from build123d import *

# Parameters (mm, degrees)
BOSS_EXTRUDE2_DEPTH          = 12
BOSS_EXTRUDE3_START          = -2
BOSS_EXTRUDE3_DEPTH          = 10
BOSS_EXTRUDE4_START          = 10
BOSS_EXTRUDE4_DEPTH          = 22
BOSS_EXTRUDE7_DEPTH          = 40
BOSS_EXTRUDE17_DEPTH         = 6
BOSS_EXTRUDE17_DEPTH_BACK    = 6
CUT_EXTRUDE_THIN1_DEPTH      = 297.279628574
CUT_EXTRUDE_THIN1_DEPTH_BACK = 297.279628574
CUT_EXTRUDE1_START           = -8
SKETCH6_R                    = 5
CUT_EXTRUDE1_DEPTH           = 231.29743947
SKETCH6_4_R                  = 2.75
CUT_EXTRUDE2_DEPTH           = 239.29743947


with BuildPart() as part:
    # Sketch2 → Boss-Extrude2 (new body)
    with BuildSketch(Plane(origin=(0, 0, 0), x_dir=(1, 0, 0), z_dir=(0, 1, 0))):
        with BuildLine():
            Line((-292.596610314, 15.743442535), (-276.02456554, 0))
            Line((-276.02456554, 0), (-292.596610314, -17.444257657))
            Line((-292.596610314, -17.444257657), (-286.510767905, -23.850407561))
            Line((-286.510767905, -23.850407561), (-256.02456554, -12.789688675))
            Line((-256.02456554, -12.789688675), (0.21086679, -12.5))
            ThreePointArc((0.21086679, -12.5), (0.401744327, -17.25142014), (0.653571446, -22))
            Line((0.653571446, -22), (6.263616969, -22))
            ThreePointArc((6.263616969, -22), (5.6, 0), (6.263616969, 22))
            Line((6.263616969, 22), (0.653571446, 22))
            ThreePointArc((0.653571446, 22), (0.401744327, 17.25142014), (0.21086679, 12.5))
            Line((0.21086679, 12.5), (-256.02456554, 12.210311325))
            Line((-256.02456554, 12.210311325), (-286.510767905, 22.149592439))
            Line((-286.510767905, 22.149592439), (-292.596610314, 15.743442535))
        make_face()
    extrude(amount=-BOSS_EXTRUDE2_DEPTH)

    # Sketch2<5> → Boss-Extrude3 (add)
    with BuildSketch(Plane(origin=(0, 0, 0), x_dir=(1, 0, 0), z_dir=(0, 1, 0)).offset(BOSS_EXTRUDE3_START)):
        with BuildLine():
            Line((25.340211435, 22), (6.263616969, 22))
            ThreePointArc((6.263616969, 22), (5.6, 0), (6.263616969, -22))
            Line((6.263616969, -22), (25.340211435, -22))
            ThreePointArc((25.340211435, -22), (24.64, 0), (25.340211435, 22))
        make_face()
    extrude(amount=-BOSS_EXTRUDE3_DEPTH)

    # Sketch2<6> → Boss-Extrude4 (add)
    with BuildSketch(Plane(origin=(0, 0, 0), x_dir=(1, 0, 0), z_dir=(0, 1, 0)).offset(BOSS_EXTRUDE4_START)):
        with BuildLine():
            ThreePointArc((0.653571446, 22), (0.401744327, 17.25142014), (0.21086679, 12.5))
            ThreePointArc((0.21086679, 12.5), (0, 0), (0.21086679, -12.5))
            ThreePointArc((0.21086679, -12.5), (0.401744327, -17.25142014), (0.653571446, -22))
            Line((0.653571446, -22), (6.263616969, -22))
            ThreePointArc((6.263616969, -22), (5.6, 0), (6.263616969, 22))
            Line((6.263616969, 22), (0.653571446, 22))
        make_face()
    extrude(amount=-BOSS_EXTRUDE4_DEPTH)

    # Sketch2<9> → Boss-Extrude7 (add)
    with BuildSketch(Plane(origin=(0, 0, 0), x_dir=(1, 0, 0), z_dir=(0, 1, 0))):
        Polygon((-292.596610314, 15.743442535), (-276.02456554, 0), (-292.596610314, -17.444257657), (-286.510767905, -23.850407561), (-219.731467486, 0.377833809), (-286.510767905, 22.149592439), align=None)
    extrude(amount=BOSS_EXTRUDE7_DEPTH)

    # Sketch4 → Boss-Extrude17 (add, two sides: drawn at the far end of the back side and taken through both)
    with BuildSketch(Plane.XY.offset(-BOSS_EXTRUDE17_DEPTH_BACK)):
        Polygon((0.653571446, 10), (-256.02456554, 40), (-256.02456554, 0), (0.653571446, 0), align=None)
    extrude(amount=BOSS_EXTRUDE17_DEPTH + BOSS_EXTRUDE17_DEPTH_BACK)

    # Sketch5 → Cut-Extrude-Thin1 (cut, two sides: drawn at the far end of the back side and taken through both)
    with BuildSketch(Plane.XY.offset(-CUT_EXTRUDE_THIN1_DEPTH_BACK)):
        Polygon((0.653571446, 10), (-256.02456554, 40), (-254.863688753, 49.932389697), (1.814448233, 19.932389697), align=None)
    extrude(amount=CUT_EXTRUDE_THIN1_DEPTH + CUT_EXTRUDE_THIN1_DEPTH_BACK, mode=Mode.SUBTRACT)

    # Sketch6 → Cut-Extrude1 (cut, through all)
    with BuildSketch(Plane(origin=(-145.085185566, 0, -137.830926288), x_dir=(-0.6887494619146907, 0, 0.724999433594416), z_dir=(-0.724999433594416, 0, -0.6887494619146907)).offset(CUT_EXTRUDE1_START)):
        with Locations((200.111770991, 29)):
            Circle(SKETCH6_R)
        with Locations((200.111770991, -1)):
            Circle(SKETCH6_R)
    cut_extrude1 = extrude(amount=-CUT_EXTRUDE1_DEPTH, mode=Mode.SUBTRACT)

    # Sketch6<4> → Cut-Extrude2 (cut, symmetric)
    with BuildSketch(Plane(origin=(-145.085185566, 0, -137.830926288), x_dir=(-0.6887494619146907, 0, 0.724999433594416), z_dir=(-0.724999433594416, 0, -0.6887494619146907))):
        with Locations((200.111770991, 29)):
            Circle(SKETCH6_4_R)
        with Locations((200.111770991, -1)):
            Circle(SKETCH6_4_R)
    cut_extrude2 = extrude(amount=CUT_EXTRUDE2_DEPTH, both=True, mode=Mode.SUBTRACT)

    # Mirror1: Cut-Extrude1, Cut-Extrude2 across plane
    add(cut_extrude1.mirror(Plane.XY), mode=Mode.SUBTRACT)
    add(cut_extrude2.mirror(Plane.XY), mode=Mode.SUBTRACT)


solid = part.part
CAD build for the part. Positions are in the model's coordinates, mm. A direction names the side the tool comes from. Coordinates: 2 decimals unless noted, no trailing zeros. Loops run counter-clockwise (first coordinate to the right, second up) from the corner with the lowest first, then second, coordinate; pieces in that order, holes last. Notation, with made-up numbers: (8.25, 5) - (66.25, 5) arc R14 cw to (66.25, 21) - close; hole circle Ø11 at (-25.5, 24). An arc over 180 degrees is marked (long way). Write item = value, one per line. Start each with the question number.
Q1. Flat gauge pins, fed straight in: pin 1 Ø8 at (y, z) = (2, 10.5) entering from -X; pin 2 Ø10 at (x, z) = (15, -10) entering from +Y; pin 3 Ø8 at (y, z) = (11.5, 6.5) entering from -X. Where does each tip first touch, or does it go through?
Q2. Which spindle directions (+Z, -Z, +X, -X, +Y, -Y) get a long thin tool onto all of the face, cutting with end or side? Do faces 1 (the flat face through (-130, 0, -9)), 2 (the flat face through (-278.594, -3.152, -14.32)), 3 (the flat face through (10, -6, 22)). Say none if no direction does.
Q3. Cut at B-B, the plane x = -128.5. List the corners of the cut face in (y, z).
Q4. Cut at A-A, the plane y = 17.5. List the corners of the cut face in (x, z).
Q5. Pull direction Z, two halves, no side cores. Call faces 4 (the flat face through (-289.6, 13.6, 20.6)), 5 (the flat face through (-130, 0, 9)), 6 (the cylindrical face through (-270.734, -0.78, 11.93)): pulls with the +Z half, pulls with the -Z half, needs draft (parallel to the pull), parting line crosses it, or undercut.
Q6. Drill centre lines: L1, parallel to Z at x = 10, y = -10; L2, parallel to Y at x = -138, z = -5; L3, parallel to Z at x = -33.5, y = 11.5. Where is each one in solid material? Low to high.
Q7. Cut at C-C, the plane x = -73. List the corners of the cut face in (y, z), then the cut area to 3 significant figures.
Computed:
q1.pin_1 = -289.8
q1.pin_2 = -2
q1.pin_3 = -286
q2.face_1 = -Z, +Y
q2.face_2 = none
q2.face_3 = +Z, +X, +Y, -Y
q3.outline = (-12, -12.35) - (0, -12.35) - (0, -6) - (25.1, -6) - (25.1, 6) - (0, 6) - (0, 12.65) - (-12, 12.65) - close
q4.outline = (-292.6, -15.74) - (-286.51, -22.15) - (-236.98, -6) - (-63.52, -6) - (-63.52, 6) - (-237.31, 6) - (-286.51, 23.85) - (-292.6, 17.44) - (-276.02, 0) - close
q5.face_4 = pulls with the +Z half
q5.face_5 = needs draft
q5.face_6 = undercut
q6.L1 = -22 to 22
q6.L2 = -12 to 26.21
q6.L3 = -6 to 6
q7.outline = (-12, -12.42) - (0, -12.42) - (0, -6) - (18.61, -6) - (18.61, 6) - (0, 6) - (0, 12.58) - (-12, 12.58) - close
q7.area = 523 mm²
